from build123d import *

# Parameters (mm, degrees)
CROQUIS1_R              = 20
CROQUIS1_R_2            = 8
SALIENTE_EXTRUIR1_DEPTH = 5
CROQUIS2_R              = 25
CROQUIS2_R_2            = 8
SALIENTE_EXTRUIR2_DEPTH = 3


with BuildPart() as part:
    # Croquis1 → Saliente-Extruir1 (new, symmetric)
    with BuildSketch(Plane.XY):
        Circle(CROQUIS1_R)
        Circle(CROQUIS1_R_2, mode=Mode.SUBTRACT)
    extrude(amount=SALIENTE_EXTRUIR1_DEPTH, both=True)

    # Croquis2 → Saliente-Extruir2 (add)
    with BuildSketch(Plane.XY.offset(5)):
        Circle(CROQUIS2_R)
        Circle(CROQUIS2_R_2, mode=Mode.SUBTRACT)
    saliente_extruir2 = extrude(amount=SALIENTE_EXTRUIR2_DEPTH)

    # Simetría1: Saliente-Extruir2 across plane
    add(saliente_extruir2.mirror(Plane.XY))


solid = part.part
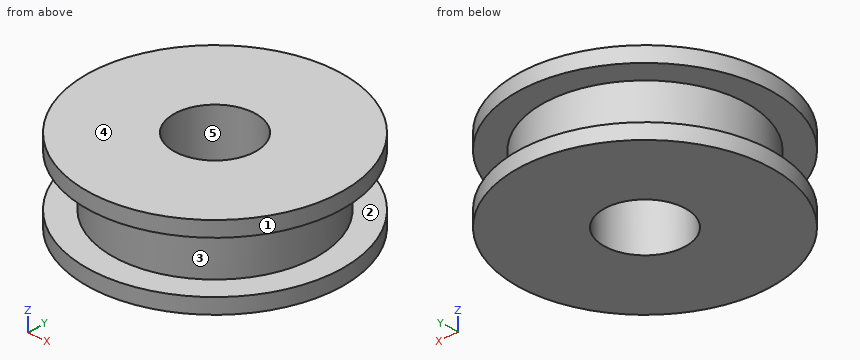
Design review of the part built by this model. Coordinates are the model's own, in mm. Face numbers are marked on the shaded views. A direction names the side the tool comes from. Coordinates: 2 decimals unless noted, no trailing zeros. Order: outer loops, then holes, each group sorted by start corner. A loop starts at its lowest first (then second) coordinate and runs counter-clockwise, first axis right, second up. Notation, with made-up numbers: (51.25, 64) -> (67.25, 64) arc R29 ccw to (67.25, 98) -> close; hole circle Ø4 at (14, 47.5). An arc over 180 degrees is marked (long way). Use one line per item in the form item = value. Start each with the question number.
(1) Add section C-C on z = -2. State the section outline as (x, y) points.
(2) For probe 1 along Z at (x, y) = (-19.5, 10); probe 2 along Y at (x, z) = (0, 1.5); probe 3 along Y at (x, z) = (6.5, -7), list the stretches that pass through material, from the lowest coordinate up.
(3) For the marked faces 1 and 2, list the 3-axis set-ups (+Z, -Z, +X, -X, +Y, -Y) from which the entire face can be reached by the end or side of a thin tool; tool diameter is ignored.
(4) Add section A-A on y = 0. State the section outline as (x, z) points, plus the area to 3 significant figures.
(5) Insertion check: pin 1 (5 mm diameter, centred on x = 12.5, z = -4.5, fed in from -Y); pin 2 (1 mm diameter, centred on x = -7.5, z = 1, fed in from +Y) (3 decimals); pin 3 (2 mm diameter, centred on x = 5, y = -0.5, fed in from +Z); pin 4 (1.5 mm diameter, centred on y = 14.5, z = -2.5, fed in from -X). Each pin has a flat end and moves straight along its axis. Give the tip position at first contact, or say it passes through.
(6) Add section D-D on x = -18.5. State the section outline as (y, z) points.
(7) The part is to be moulded in two halves that separate along X. For the marked faces 3, 4 and 5, say which applies: +X half, -X half, draft (parallel to the pull), parting line (faces both ways), or undercut.
Answer block:
q1.outline = circle Ø40 at (0, 0); hole circle Ø16 at (0, 0)
q2.probe_1 = -8 to -5, 5 to 8
q2.probe_2 = -20 to -8, 8 to 20
q2.probe_3 = -24.14 to -4.66, 4.66 to 24.14
q3.face_1 = +Z, -Z
q3.face_2 = none
q4.outline = (-25, -8) -> (-8, -8) -> (-8, 8) -> (-25, 8) -> (-25, 5) -> (-20, 5) -> (-20, -5) -> (-25, -5) -> close; (8, -8) -> (25, -8) -> (25, -5) -> (20, -5) -> (20, 5) -> (25, 5) -> (25, 8) -> (8, 8) -> close
q4.area = 444 mm²
q5.pin_1 = -22.89
q5.pin_2 = 18.735
q5.pin_3 = through
q5.pin_4 = -14.52
q6.outline = (-16.82, -8) -> (16.82, -8) -> (16.82, -5) -> (7.6, -5) -> (7.6, 5) -> (16.82, 5) -> (16.82, 8) -> (-16.82, 8) -> (-16.82, 5) -> (-7.6, 5) -> (-7.6, -5) -> (-16.82, -5) -> close
q7.face_3 = parting line
q7.face_4 = draft
q7.face_5 = undercut
